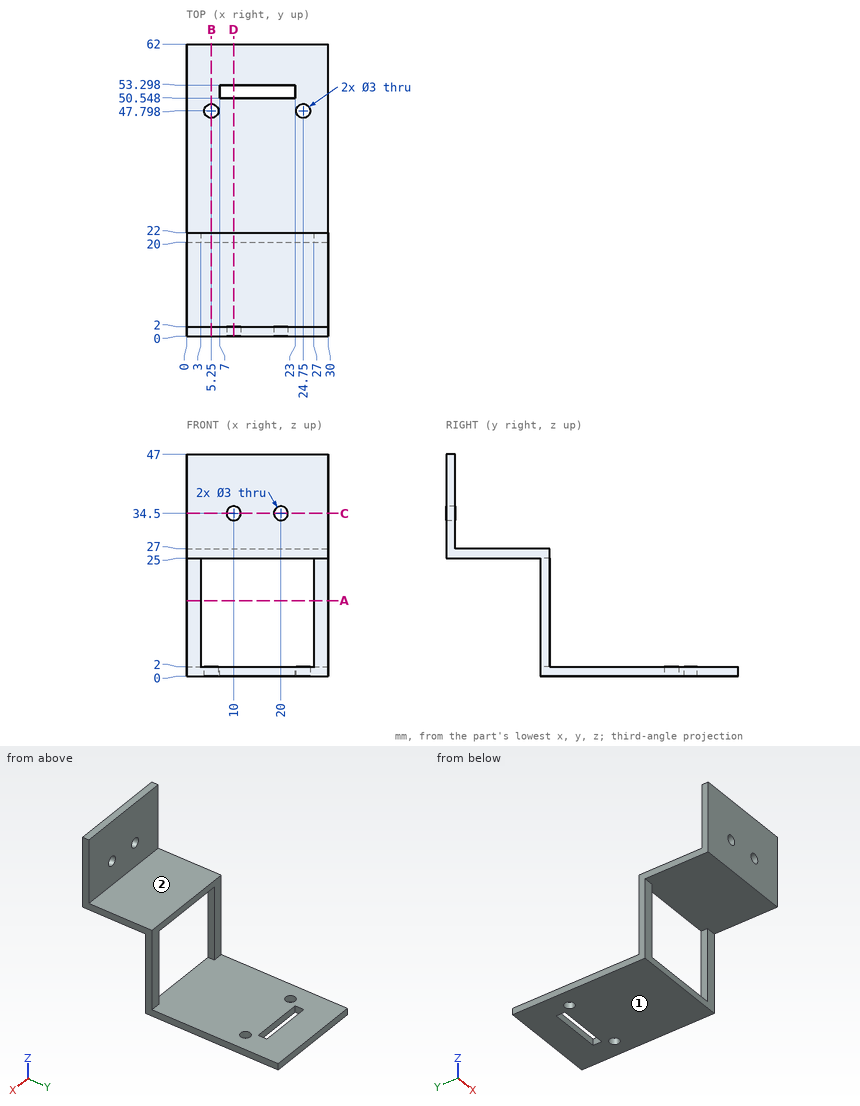
Print and shaded views of the part. All mm, measured from the part's lowest x, y and z. A direction names the side the tool comes from. Coordinates: 2 decimals unless noted, no trailing zeros. Loops run counter-clockwise (first coordinate to the right, second up) from the corner with the lowest first, then second, coordinate; pieces in that order, holes last. Notation, with made-up numbers: (16, 47.5) -> (31, 47.5) arc R20 ccw to (31, 56.5) -> close; hole circle Ø4 at (35.25, 31). An arc over 180 degrees is marked (long way). Use one line per item in the form item = value. Start each with the question number.
(1) Cut at B-B on x = 5.25. Give the cut face in (y, z), and give its area (3 significant figures).
(2) Probe probe 1 along Z at (x, y) = (17, 21); probe 2 along Y at (x, z) = (24.75, 1.35); probe 3 along Y at (x, z) = (7.5, 33.5). List the from-to ranges inside material, lowest first. Write a range as from..to.
(3) Cut at D-D on x = 10. Give the cut face in (y, z).
(4) Cut at A-A on z = 16. Give the cut face in (x, y).
(5) Flat gauge pins, fed straight in: pin 1 (3.5 mm diameter, centred on x = 24.75, y = 47.8, fed in from -Z); pin 2 (3.5 mm diameter, centred on x = 10, z = 34.5, fed in from +Y); pin 3 (6.5 mm diameter, centred on x = 8.5, y = 16, fed in from -Z); pin 4 (6 mm diameter, centred on x = 17, y = 8, fed in from +Z). Where does each tip first touch, or does it go through?
(6) Cut at C-C on z = 34.5. Give the cut face in (x, y).
(7) Tool access for the marked faces 1 and 2: list every direction of +Z, -Z, +X, -X, +Y, -Y with a clear straight run to the whole face (end or side of a thin tool).
Values:
q1.outline = (0, 25) -> (22, 25) -> (22, 27) -> (2, 27) -> (2, 47) -> (0, 47) -> close; (20, 0) -> (46.3, 0) -> (46.3, 2) -> (20, 2) -> close; (49.3, 0) -> (62, 0) -> (62, 2) -> (49.3, 2) -> close
q1.area = 162 mm2
q2.probe_1 = 0..2, 25..27
q2.probe_2 = 20..46.3, 49.3..62
q2.probe_3 = 0..2
q3.outline = (0, 25) -> (22, 25) -> (22, 27) -> (2, 27) -> (2, 33) -> (0, 33) -> close; (0, 36) -> (2, 36) -> (2, 47) -> (0, 47) -> close; (20, 0) -> (50.55, 0) -> (50.55, 2) -> (20, 2) -> close; (53.3, 0) -> (62, 0) -> (62, 2) -> (53.3, 2) -> close
q4.outline = (0, 20) -> (3, 20) -> (3, 22) -> (0, 22) -> close; (27, 20) -> (30, 20) -> (30, 22) -> (27, 22) -> close
q5.pin_1 = 0
q5.pin_2 = 2
q5.pin_3 = 25
q5.pin_4 = 27
q6.outline = (0, 0) -> (8.5, 0) -> (8.5, 2) -> (0, 2) -> close; (11.5, 0) -> (18.5, 0) -> (18.5, 2) -> (11.5, 2) -> close; (21.5, 0) -> (30, 0) -> (30, 2) -> (21.5, 2) -> close
q7.face_1 = -Z, +X, -X, +Y, -Y
q7.face_2 = +Z, +X, -X, +Y
